Part model, mm, in its own coordinate system. Face numbers are marked on the shaded views. Round coordinates to 2 decimals unless told otherwise and drop trailing zeros. Order: outer loops, then holes, each group sorted by start corner. A loop starts at its lowest first (then second) coordinate and runs counter-clockwise, first axis right, second up. Notation, with made-up numbers: (25.25, -27) -> (52.25, -27) arc R26 cw to (52.25, 12) -> close; hole circle Ø2 at (35, 9). An arc over 180 degrees is marked (long way). Answer as a JSON object with one key per item and string values. Group by question number.
```python
from build123d import *

# Parameters (mm, degrees)
SKETCH1_W           = 58
SKETCH1_H           = 40
SKETCH1_R           = 10
BOSS_EXTRUDE1_DEPTH = 9
SKETCH2_W           = 41
SKETCH2_H           = 40
CUT_EXTRUDE1_DEPTH  = 4.5
SKETCH3_R           = 1.5
CUT_EXTRUDE2_DEPTH  = 51.219518118


with BuildPart() as part:
    # Sketch1 → Boss-Extrude1 (new body)
    with BuildSketch(Plane.XY):
        Rectangle(SKETCH1_W, SKETCH1_H)
        with Locations((0, 2)):
            Circle(SKETCH1_R, mode=Mode.SUBTRACT)
    extrude(amount=BOSS_EXTRUDE1_DEPTH)

    # Sketch2 → Cut-Extrude1 (cut)
    with BuildSketch(Plane(origin=(0, 0, 0), x_dir=(-1, 0, 0), z_dir=(0, 0, -1))):
        Rectangle(SKETCH2_W, SKETCH2_H)
    extrude(amount=-CUT_EXTRUDE1_DEPTH, mode=Mode.SUBTRACT)

    # Sketch3 → Cut-Extrude2 (cut, through all)
    with BuildSketch(Plane(origin=(0, 20, 0), x_dir=(1, 0, 0), z_dir=(0, 1, 0))):
        with Locations(Location((24.75, -4.5, 0), (0, 0, 270))):
            Circle(SKETCH3_R)
        with Locations(Location((-24.75, -4.5, 0), (0, 0, 270))):
            Circle(SKETCH3_R)
    extrude(amount=-CUT_EXTRUDE2_DEPTH, mode=Mode.SUBTRACT)


solid = part.part
```
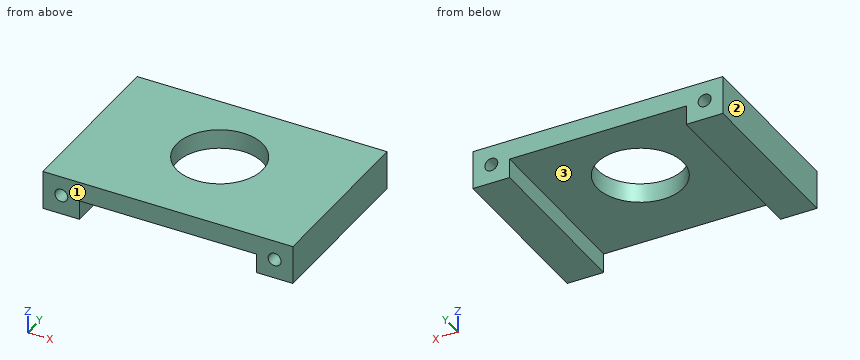
Q1. Drop a flat-ended pin along its axis: pin 1 Ø10 at (x, y) = (-14, -13.5) entering from -Z. Give the stop position or say it passes through.
Q2. Band-saw the part on A-A (x = 0). List the corners of the cut face in (y, z), plus the area to 3 significant figures.
Q3. Band-saw the part on B-B (y = 11). List the corners of the cut face in (x, z), plus the area to 3 significant figures.
Q4. Two-plate mould, pull along X, no slides. Class the marked faces 1, 2 and 3: +X half, -X half, draft (parallel to the pull), parting line (faces both ways), or undercut.
Q5. Wall check: line 1 (X direction, y = 2, z = 6.9); line 2 (X direction, y = -5, z = 0.75); line 3 (X direction, y = 7.5, z = 5). Give the ranges that are in metal, low to high. Write a range as [from, to].
Q6. Band-saw the part on C-C (z = 1.5). List the corners of the cut face in (x, y), plus the area to 3 significant figures.
Q7. Band-saw the part on D-D (z = 7.5). List the corners of the cut face in (x, y), plus the area to 3 significant figures.
Completed:
{
 "1": {"pin 1": "z = 4.5"},
 "2": {"outline": "(-20, 4.5) -> (-8, 4.5) -> (-8, 9) -> (-20, 9) -> close; (12, 4.5) -> (20, 4.5) -> (20, 9) -> (12, 9) -> close", "area": "90.0 mm2"},
 "3": {"outline": "(-29, 0) -> (-20.5, 0) -> (-20.5, 4.5) -> (-4.36, 4.5) -> (-4.36, 9) -> (-29, 9) -> close; (4.36, 4.5) -> (20.5, 4.5) -> (20.5, 0) -> (29, 0) -> (29, 9) -> (4.36, 9) -> close; hole circle Ø3 at (-24.75, 4.5); hole circle Ø3 at (24.75, 4.5)", "area": "284 mm2"},
 "4": {"face 1": "draft", "face 2": "-X half", "face 3": "undercut"},
 "5": {"line 1": "[-29, -10], [10, 29]", "line 2": "[-29, -20.5], [20.5, 29]", "line 3": "[-29, -26.16], [-23.34, -8.35], [8.35, 23.34], [26.16, 29]"},
 "6": {"outline": "(-29, -20) -> (-20.5, -20) -> (-20.5, 20) -> (-29, 20) -> close; (20.5, -20) -> (29, -20) -> (29, 20) -> (20.5, 20) -> close", "area": "680 mm2"},
 "7": {"outline": "(-29, -20) -> (29, -20) -> (29, 20) -> (-29, 20) -> close; hole circle Ø20 at (0, 2)", "area": "2,010 mm2"}
}
